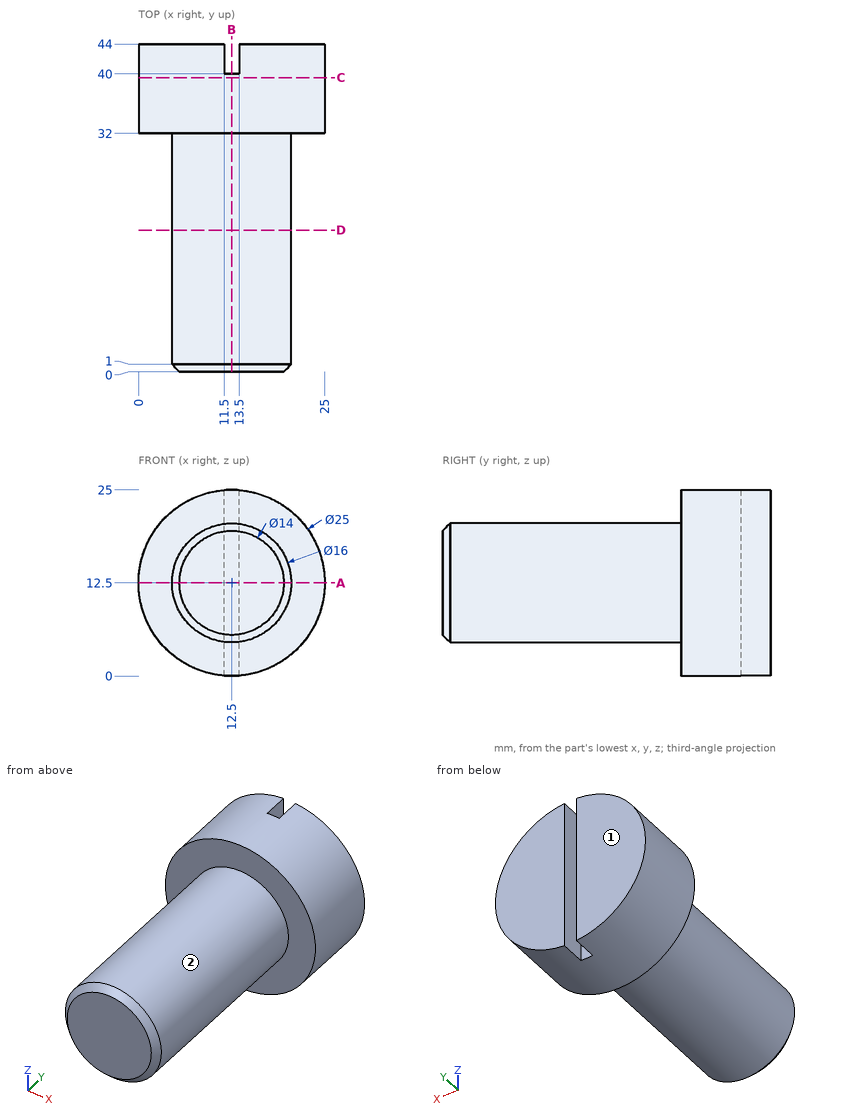
Geometry check sheet. Reference: drawing and pictorial views, mm from the part's lowest x, y, z. A direction names the side the tool comes from. Coordinates: 2 decimals unless noted, no trailing zeros. Order: outer loops, then holes, each group sorted by start corner. A loop starts at its lowest first (then second) coordinate and runs counter-clockwise, first axis right, second up. Notation, with made-up numbers: (43.5, -9) -> (72.5, -9) arc R32 ccw to (72.5, 18) -> close; hole circle Ø2 at (-23, 37). An arc over 180 degrees is marked (long way). Put each result on its own line as item: value. Start each with the question number.
1) Tool access check on the marked faces 1 and 2. Record the directions out of +Z, -Z, +X, -X, +Y, -Y that give a thin tool (end or side, any length) a straight path to the whole face; none if there is none.
2) Material ranges on L1, parallel to Y at x = 21.75, z = 11.5; L2, parallel to X at y = 41, z = 21; L3, parallel to X at y = 36.5, z = 17.75, recorded low to high.
3) Cross-section at B-B (x = 12.5). Enter the section's corners in (y, z).
4) Cross-section at C-C (y = 39.5). Enter the section's corners in (x, z), plus the area to 3 significant figures.
5) Go/stop test with flat-tipped pins: pin 1 (3 mm diameter, centred on y = 35, z = 10, fed in from +X); pin 2 (4.5 mm diameter, centred on y = 41, z = 9.5, fed in from -X); pin 3 (1.2 mm diameter, centred on y = 43, z = 7, fed in from +X). Record where each tip stops, or that it passes through.
6) Cross-section at A-A (z = 12.5). Enter the section's corners in (x, y), plus the area to 3 significant figures.
7) Cross-section at D-D (y = 19). Enter the section's corners in (x, z), plus the area to 3 significant figures.
Geometry check:
1. face 1: +Z, -Z, +X, -X, +Y
1. face 2: -Y
2. L1: y = 32 to 44
2. L2: x = 3.33 to 11.5, 13.5 to 21.67
2. L3: x = 1.16 to 23.84
3. outline: (0, 5.5) -> (1, 4.5) -> (32, 4.5) -> (32, 0) -> (40, 0) -> (40, 25) -> (32, 25) -> (32, 20.5) -> (1, 20.5) -> (0, 19.5) -> close
4. outline: circle Ø25 at (12.5, 12.5)
4. area: 491 mm^2
5. pin 1: stops at x = 24.96
5. pin 2: stops at x = 0.02
5. pin 3: stops at x = 24
6. outline: (0, 32) -> (4.5, 32) -> (4.5, 1) -> (5.5, 0) -> (19.5, 0) -> (20.5, 1) -> (20.5, 32) -> (25, 32) -> (25, 44) -> (13.5, 44) -> (13.5, 40) -> (11.5, 40) -> (11.5, 44) -> (0, 44) -> close
6. area: 803 mm^2
7. outline: circle Ø16 at (12.5, 12.5)
7. area: 201 mm^2
